Job drawing, mm, ordinate dimensions from the low corner. One solid piece. Coordinates: 2 decimals unless noted, no trailing zeros. Write each loop counter-clockwise with the first axis right and the second up, starting at its lowest first coordinate (ties: lowest second). Pieces come first, ordered by that corner, then holes. Notation, with made-up numbers: (64, -28) -> (82, -28) arc R15 cw to (82, -11) -> close; hole circle Ø1 at (65.5, 8). An arc over 180 degrees is marked (long way). Answer as a JSON object with one key per item and string values. Group by question number.
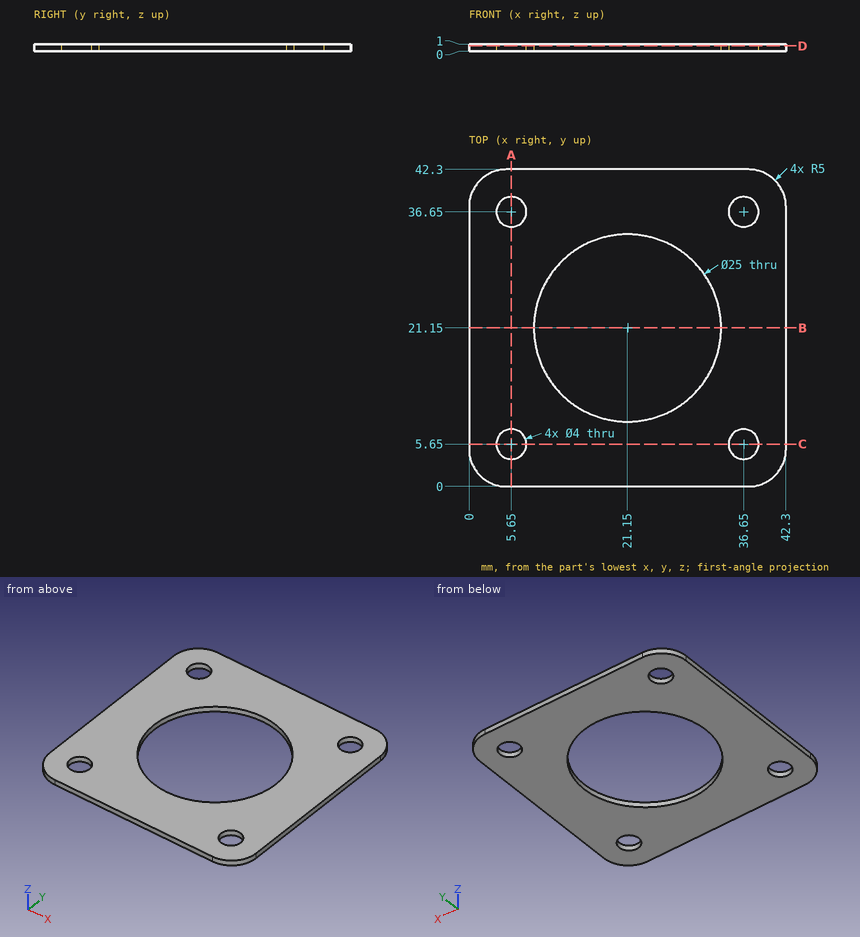
(1) Cut at B-B on y = 21.15. List the corners of the cut face in (x, z), plus the area to 3 significant figures.
(2) Wall check: probe 1 along Y at (x, z) = (36.65, 0.85); probe 2 along Y at (x, z) = (7, 0.55); probe 3 along X at (y, z) = (6.5, 0.65). Give the ranges that are in metal, low to high.
(3) Cut at A-A on x = 5.65. List the corners of the cut face in (y, z).
(4) Cut at D-D on z = 0.75. List the corners of the cut face in (x, y), plus the area to 3 significant figures.
(5) Pin check, flat tip, straight feed: pin 1 (8 mm diameter, centred on x = 17.5, y = 11, fed in from -Z). Stop position of the tip, or through.
Results found:
{
 "1": {"outline": "(0, 0) -> (8.65, 0) -> (8.65, 1) -> (0, 1) -> close; (33.65, 0) -> (42.3, 0) -> (42.3, 1) -> (33.65, 1) -> close", "area": "17.3 mm²"},
 "2": {"probe 1": "y = 0 to 3.65, 7.65 to 34.65, 38.65 to 42.3", "probe 2": "y = 0 to 4.17, 7.13 to 35.17, 38.13 to 42.3", "probe 3": "x = 0 to 3.84, 7.46 to 34.84, 38.46 to 42.3"},
 "3": {"outline": "(0, 0) -> (3.65, 0) -> (3.65, 1) -> (0, 1) -> close; (7.65, 0) -> (34.65, 0) -> (34.65, 1) -> (7.65, 1) -> close; (38.65, 0) -> (42.3, 0) -> (42.3, 1) -> (38.65, 1) -> close"},
 "4": {"outline": "(0, 5) arc R5 ccw to (5, 0) -> (37.3, 0) arc R5 ccw to (42.3, 5) -> (42.3, 37.3) arc R5 ccw to (37.3, 42.3) -> (5, 42.3) arc R5 ccw to (0, 37.3) -> close; hole circle Ø4 at (5.65, 5.65); hole circle Ø4 at (5.65, 36.65); hole circle Ø25 at (21.15, 21.15); hole circle Ø4 at (36.65, 5.65); hole circle Ø4 at (36.65, 36.65)", "area": "1,230 mm²"},
 "5": {"pin 1": "stops at z = 0"}
}
